Check sheet for the drawn part. Datum: minimum x, y, z corner. Units: mm. A direction names the side the tool comes from. Give positions to 0.01 mm unless a question says otherwise; leave off trailing zeros. Loops run counter-clockwise (first coordinate to the right, second up) from the corner with the lowest first, then second, coordinate; pieces in that order, holes last. Notation, with made-up numbers: (-34.5, -14) - (-13.5, -14) arc R10 cw to (-13.5, -7) - close; hole circle Ø2 at (89, 22.5). An arc over 180 degrees is marked (long way). Answer in a Markdown table with one row per item.
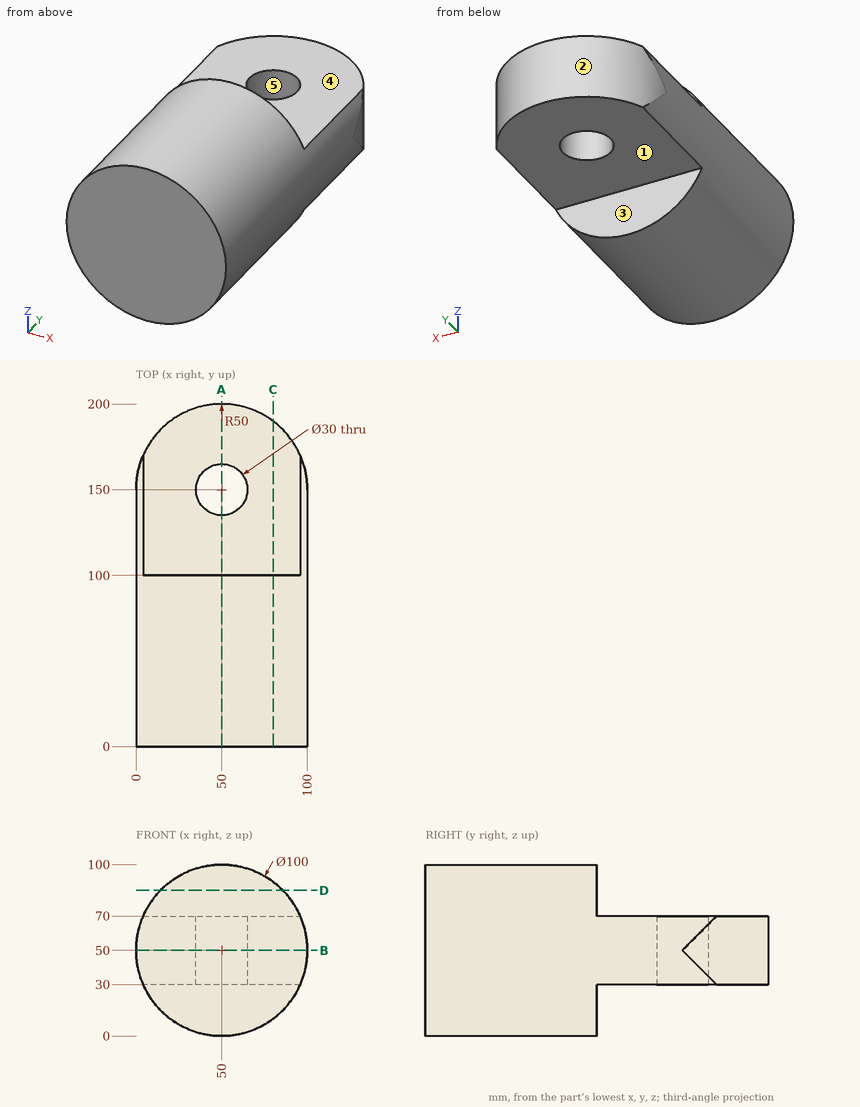
Q1. Sectioned sample at B-B (z = 50). Record the cut outline in (x, y), and give its area (3 significant figures).
Completed:
| item | result |
|---|---|
| outline | (0, 0) - (100, 0) - (100, 150) arc R50 ccw to (0, 150) - close; hole circle Ø30 at (50, 150) |
| area | 18,200 mm^2 |
Q2. Draft check along Y on the marked faces 3, 4 and 5. Enter one of: +Y half, -Y half, draft (parallel to the pull), parting line (faces both ways), or undercut.
Completed:
| item | result |
|---|---|
| face 3 | +Y half |
| face 4 | draft |
| face 5 | undercut |
Q3. Sectioned sample at C-C (x = 80). Record the cut outline in (y, z), and give its area (3 significant figures).
Completed:
| item | result |
|---|---|
| outline | (0, 10) - (100, 10) - (100, 30) - (190, 30) - (190, 70) - (100, 70) - (100, 90) - (0, 90) - close |
| area | 11,600 mm^2 |
Q4. Sectioned sample at A-A (x = 50). Record the cut outline in (y, z).
Completed:
| item | result |
|---|---|
| outline | (0, 0) - (100, 0) - (100, 30) - (135, 30) - (135, 70) - (100, 70) - (100, 100) - (0, 100) - close; (165, 30) - (200, 30) - (200, 70) - (165, 70) - close |
Q5. Go/stop test with flat-tipped pins: P1, Ø3, axis at y = 110.5, z = 30, coming from the -X side; P2, Ø5, axis at y = 28, z = 53, coming from the -X side; P3, Ø1, axis at x = 44, y = 111.5, coming from the +Z side. Record where each tip stops, or that it passes through.
Completed:
| item | result |
|---|---|
| P1 | x = 3.55 |
| P2 | x = 0 |
| P3 | z = 70 |
Q6. Sectioned sample at D-D (z = 85). Record the cut outline in (x, y), and give its area (3 significant figures).
Completed:
| item | result |
|---|---|
| outline | (14.29, 0) - (85.71, 0) - (85.71, 100) - (14.29, 100) - close |
| area | 7,140 mm^2 |
Q7. Tool access check on the marked faces 1 and 2. Record the directions out of +Z, -Z, +X, -X, +Y, -Y that give a thin tool (end or side, any length) a straight path to the whole face; none if there is none.
Completed:
| item | result |
|---|---|
| face 1 | -Z, +X, -X, +Y |
| face 2 | +Z, -Z, +Y |
Q8. Thickness scan on line 1 (Z direction, x = 80.5, y = 119.5); line 2 (Y direction, x = 58, z = 20); line 3 (X direction, y = 8, z = 79.5). Record the ranges inside material, lowest first.
Completed:
| item | result |
|---|---|
| line 1 | 30 to 70 |
| line 2 | 0 to 100 |
| line 3 | 9.63 to 90.37 |
